Drawing for the job (mm, zero at the part's lowest x, y, z). A direction names the side the tool comes from. Round coordinates to 2 decimals unless told otherwise and drop trailing zeros. Write each loop counter-clockwise with the first axis right and the second up, starting at its lowest first coordinate (ties: lowest second). Pieces come first, ordered by that corner, then holes.
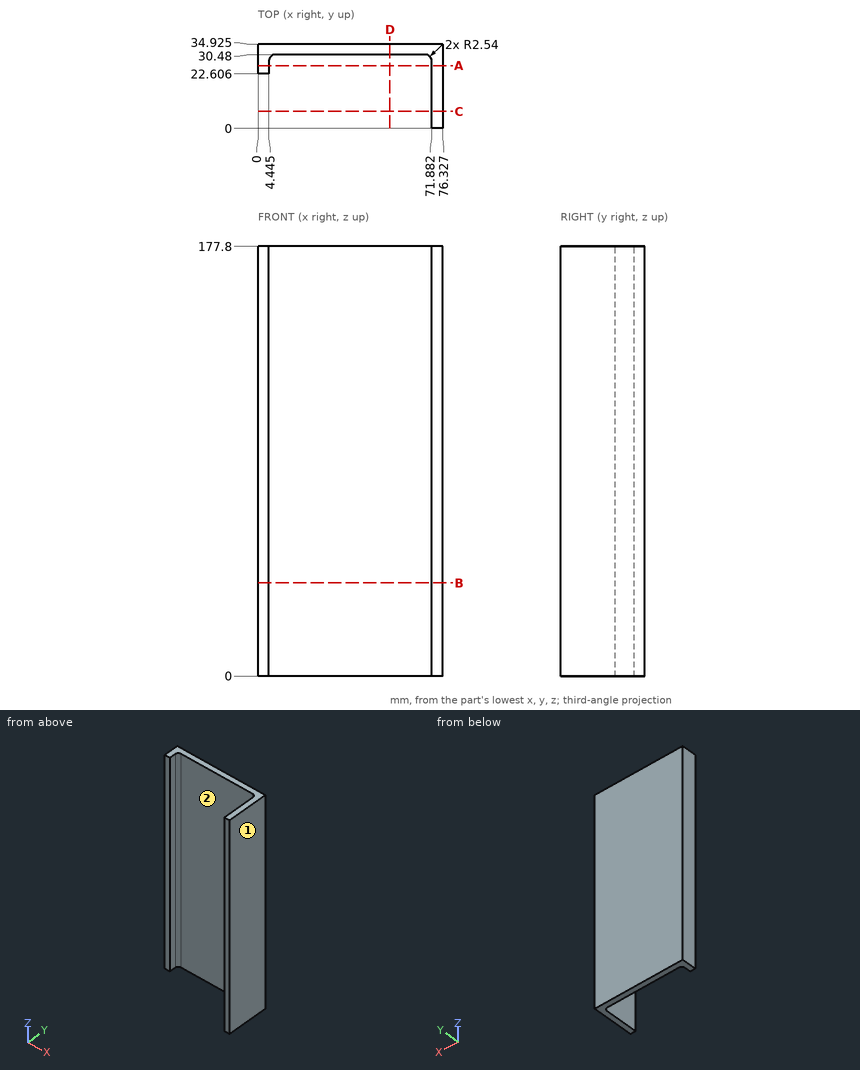
Q1. Saw through at B-B, the plane z = 38.5. Write the cut outline in (x, y) (3 decimals).
Q2. Saw through at A-A, the plane y = 26. Write the cut outline in (x, z) (3 decimals).
Q3. Wall check: line 1 (Y direction, x = 44, z = 169) (3 decimals); line 2 (X direction, y = 20, z = 92.5); line 3 (X direction, y = 30, z = 95). Give the ranges that are in metal, low to high.
Q4. Saw through at D-D, the plane x = 54.5. Write the cut outline in (y, z) (3 decimals).
Q5. Saw through at C-C, the plane y = 7. Write the cut outline in (x, z).
Q6. Tool access for the marked faces 1 and 2: list every direction of +Z, -Z, +X, -X, +Y, -Y with a clear straight run to the whole face (end or side of a thin tool).
Q7. Drop flat-ended pins along their axis: P1, Ø12, axis at x = 20, z = 85, coming from the -Y side; P2, Ø10, axis at x = 10.5, z = 116, coming from the -Y side; P3, Ø1.3, axis at x = 3, z = 57, coming from the -Y side. Give the stop position or say it passes through.
Computed:
1. outline: (0, 22.606) - (4.445, 22.606) - (4.445, 27.94) arc R2.54 cw to (6.985, 30.48) - (69.342, 30.48) arc R2.54 cw to (71.882, 27.94) - (71.882, 0) - (76.327, 0) - (76.327, 34.925) - (0, 34.925) - close
2. outline: (0, 0) - (4.445, 0) - (4.445, 177.8) - (0, 177.8) - close; (71.882, 0) - (76.327, 0) - (76.327, 177.8) - (71.882, 177.8) - close
3. line 1: y = 30.48 to 34.925
3. line 2: x = 71.88 to 76.33
3. line 3: x = 0 to 5.5, 70.83 to 76.33
4. outline: (30.48, 0) - (34.925, 0) - (34.925, 177.8) - (30.48, 177.8) - close
5. outline: (71.88, 0) - (76.33, 0) - (76.33, 177.8) - (71.88, 177.8) - close
6. face 1: +Z, -Z, +X, +Y, -Y
6. face 2: +Z, -Z, -Y
7. P1: stops at y = 30.48
7. P2: stops at y = 30
7. P3: stops at y = 22.61
